CAD build for the part. Positions are in the model's coordinates, mm. Face numbers are marked on the shaded views. Coordinates: 2 decimals unless noted, no trailing zeros. Order: outer loops, then holes, each group sorted by start corner. A loop starts at its lowest first (then second) coordinate and runs counter-clockwise, first axis right, second up. Notation, with made-up numbers: (-39, -27) - (-7, -27) arc R17 ccw to (-7, -1) - close; hole circle Ø5 at (51, 18.25). An arc over 180 degrees is marked (long way). Return JSON: item names as keys, results as strings.
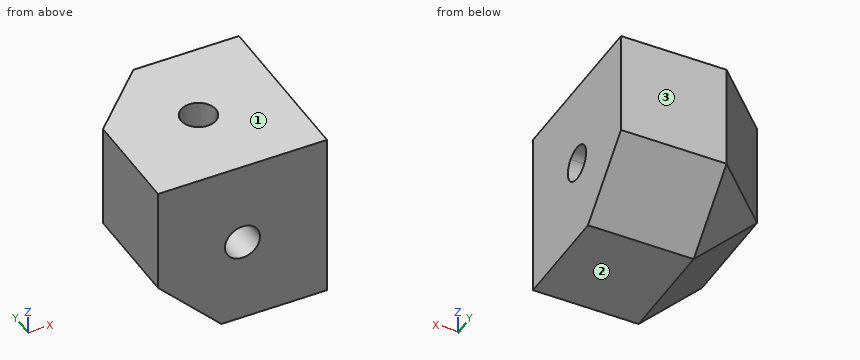
from build123d import *

# Parameters (mm, degrees)
F0_W     = 40
F0_H     = 40
F1_DEPTH = 40
F3_DEPTH = 16
F5_DEPTH = 16
F7_DEPTH = 16
F8_SIZE  = 15


with BuildPart() as f1:
    # F0 (on Top) → F1 (new body)
    with BuildSketch(Plane.XY):
        with Locations((20, 20)):
            Rectangle(F0_W, F0_H)
    extrude(amount=F1_DEPTH)

    # F2 (on face) → F3 (cut)
    with BuildSketch(Plane.XZ):
        with BuildLine():
            ThreePointArc((24.15, 20), (21.5881362443, 23.8341000599), (17.0655068581, 22.9344931419))
            Line((17.0655068581, 22.9344931419), (22.9344931419, 17.0655068581))
            ThreePointArc((22.9344931419, 17.0655068581), (23.8341000599, 18.4118637557), (24.15, 20))
        make_face()
        with BuildLine():
            Line((22.9344931419, 17.0655068581), (17.0655068581, 22.9344931419))
            ThreePointArc((17.0655068581, 22.9344931419), (17.0655068581, 17.0655068581), (22.9344931419, 17.0655068581))
        make_face()
    extrude(amount=-F3_DEPTH, mode=Mode.SUBTRACT)

    # F4 (on face) → F5 (cut)
    with BuildSketch(Plane.YZ.offset(40)):
        with BuildLine():
            ThreePointArc((24.15, 20), (21.5881362443, 23.8341000599), (17.0655068581, 22.9344931419))
            Line((17.0655068581, 22.9344931419), (22.9344931419, 17.0655068581))
            ThreePointArc((22.9344931419, 17.0655068581), (23.8341000599, 18.4118637557), (24.15, 20))
        make_face()
        with BuildLine():
            Line((22.9344931419, 17.0655068581), (17.0655068581, 22.9344931419))
            ThreePointArc((17.0655068581, 22.9344931419), (17.0655068581, 17.0655068581), (22.9344931419, 17.0655068581))
        make_face()
    extrude(amount=-F5_DEPTH, mode=Mode.SUBTRACT)

    # F6 (on face) → F7 (cut)
    with BuildSketch(Plane.XY.offset(40)):
        with BuildLine():
            ThreePointArc((24.15, 20), (21.5881362443, 23.8341000599), (17.0655068581, 22.9344931419))
            Line((17.0655068581, 22.9344931419), (22.9344931419, 17.0655068581))
            ThreePointArc((22.9344931419, 17.0655068581), (23.8341000599, 18.4118637557), (24.15, 20))
        make_face()
        with BuildLine():
            Line((22.9344931419, 17.0655068581), (17.0655068581, 22.9344931419))
            ThreePointArc((17.0655068581, 22.9344931419), (17.0655068581, 17.0655068581), (22.9344931419, 17.0655068581))
        make_face()
    extrude(amount=-F7_DEPTH, mode=Mode.SUBTRACT)

    # F8
    f8_edges = [f1.edges().sort_by_distance(p)[0] for p in [
        (20, 40, 0),
        (0, 20, 0),
        (0, 40, 20),
    ]]
    chamfer(f8_edges, length=F8_SIZE)


solid = f1.part
Item 1: Band-saw the part on D-D, the plane y = 28.5. List the corners of the cut face in (x, z).
Findings below:
{"outline": "(3.5, 15) - (15, 3.5) - (40, 3.5) - (40, 40) - (3.5, 40) - close"}
Item 2: Band-saw the part on B-B, the plane x = 30. List the corners of the cut face in (y, z), then the cut area to 3 significant figures.
Findings below:
{"outline": "(0, 0) - (25, 0) - (40, 15) - (40, 40) - (0, 40) - close; hole circle Ø8.3 at (20, 20)", "area": "1,430 mm²"}
Item 3: Mould opens along Z. For the marked faces 1, 2 and 3 say: released by +Z, released by -Z, zero draft, split by the parting line, or undercut.
Findings below:
{"face 1": "released by +Z", "face 2": "released by -Z", "face 3": "zero draft"}
Item 4: Wall check: L1, parallel to Z at x = 20, y = 11; L2, parallel to Z at x = 21.5, y = 22.5. Give the ranges that are in metal, low to high. Write a range as [from, to].
Findings below:
{"L1": "z = [0, 15.85], [24.15, 40]", "L2": "z = [0, 24]"}
Item 5: Band-saw the part on C-C, the plane x = 20. List the corners of the cut face in (y, z).
Findings below:
{"outline": "(0, 0) - (25, 0) - (40, 15) - (40, 40) - (24.15, 40) - (24.15, 24) - (16, 24) - (16, 15.85) - (0, 15.85) - close; (0, 24.15) - (15.85, 24.15) - (15.85, 40) - (0, 40) - close"}
Item 6: Drop flat-ended pins along their axis: P1, Ø4, axis at y = 22, z = 20, coming from the +X side; P2, Ø2, axis at x = 13, y = 29.5, coming from the -Z side; P3, Ø4, axis at x = 22, y = 19.5, coming from the +Z side. Give the stop position or say it passes through.
Findings below:
{"P1": "stops at x = 24", "P2": "stops at z = 5.09", "P3": "stops at z = 24"}
Item 7: Band-saw the part on A-A, the plane z = 25.5. List the corners of the cut face in (x, y), then the cut area to 3 significant figures.
Findings below:
{"outline": "(0, 0) - (40, 0) - (40, 40) - (15, 40) - (0, 25) - close; hole circle Ø8.3 at (20, 20)", "area": "1,430 mm²"}
